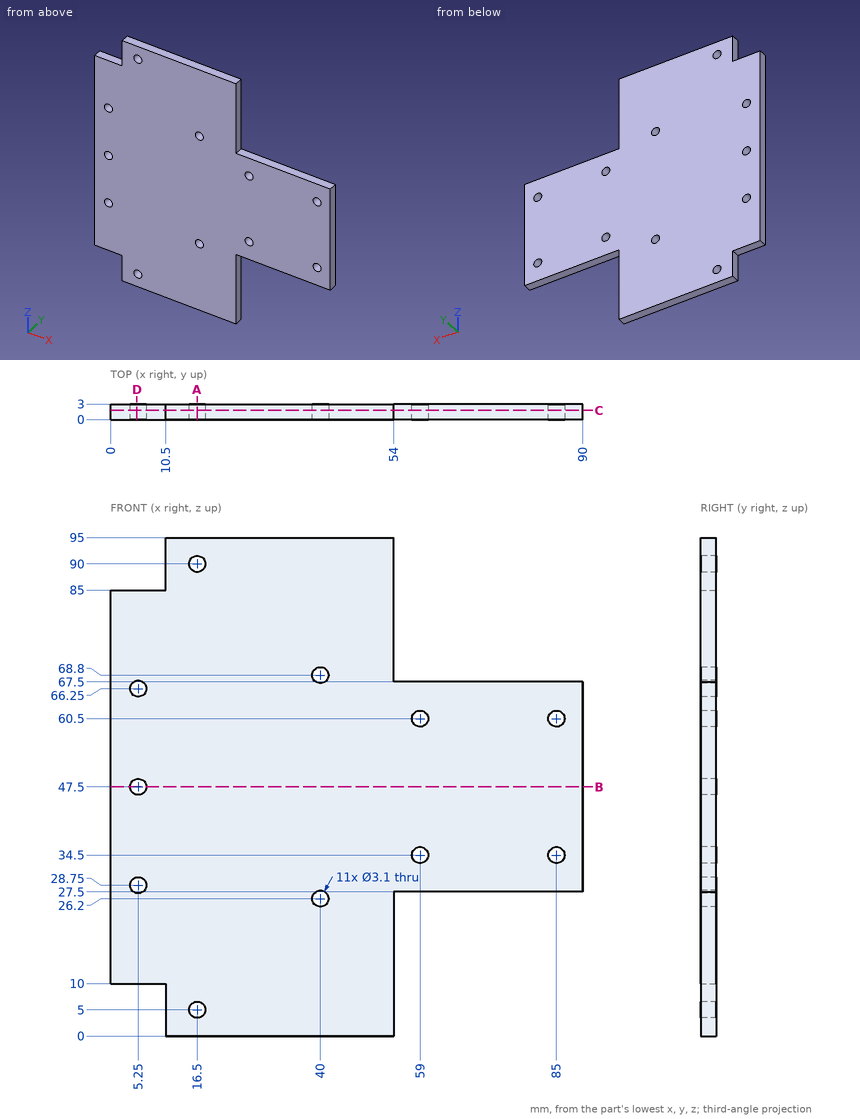
Here's the drawing with two shaded views (mm, measured from the low corner). I have some questions. Coordinates: 2 decimals unless noted, no trailing zeros. Write each loop counter-clockwise with the first axis right and the second up, starting at its lowest first coordinate (ties: lowest second). Pieces come first, ordered by that corner, then holes. Notation, with made-up numbers: M -38.5,72.25 L 0.5,72.25 A12 ccw 0.5,79.25 Z; hole C 3,76.5 d11. An arc over 180 degrees is marked long. Use one line per item in the form item = value.
Q1. If we section it at C-C (y = 1.8): State how many separate pieces and enclosed holes the cut face has, then the cut area to 3 significant figures.
Model answer:
separate_pieces = 1
enclosed_holes = 11
area = 6,280 mm^2
Q2. If we section it at D-D (x = 5): Write out the boundary of the cut face in (y, z).
Model answer:
outline = M 0,10 L 3,10 L 3,27.22 L 0,27.22 Z; M 0,30.28 L 3,30.28 L 3,45.97 L 0,45.97 Z; M 0,49.03 L 3,49.03 L 3,64.72 L 0,64.72 Z; M 0,67.78 L 3,67.78 L 3,85 L 0,85 Z
Q3. If we section it at A-A (x = 16.5): Write out the boundary of the cut face in (y, z).
Model answer:
outline = M 0,0 L 3,0 L 3,3.45 L 0,3.45 Z; M 0,6.55 L 3,6.55 L 3,88.45 L 0,88.45 Z; M 0,91.55 L 3,91.55 L 3,95 L 0,95 Z
Q4. If we section it at B-B (z = 47.5): Write out the boundary of the cut face in (x, y), then the cut area to 3 significant figures.
Model answer:
outline = M 0,0 L 3.7,0 L 3.7,3 L 0,3 Z; M 6.8,0 L 90,0 L 90,3 L 6.8,3 Z
area = 261 mm^2
Q5. I need wall thicknesses on line 1 along Z through (x, y) = (17, 0.85); line 2 along X through (y, z) = (2.2, 90); line 3 along X through (y, z) = (0.2, 29). Which ranges of each line are inside material? Lowest first, please. Write a range as from..to.
Model answer:
line_1 = 0..3.53, 6.47..88.53, 91.47..95
line_2 = 10.5..14.95, 18.05..54
line_3 = 0..3.72, 6.78..90
Q6. For P1, Ø0.9, axis at y = 1, z = 88.5, coming from the -X side, with a flat end and sliding along its axis, tell me the tip position at first contact or that it passes through.
Model answer:
P1 = 10.5
